Could you check a few things on this model? Use its own coordinates, in mm. A direction names the side the tool comes from. Coordinates: 2 decimals unless noted, no trailing zeros. Order: outer loops, then holes, each group sorted by start corner. A loop starts at its lowest first (then second) coordinate and runs counter-clockwise, first axis right, second up. Notation, with made-up numbers: (32.25, 42) -> (43.25, 42) arc R17 cw to (43.25, 71) -> close; hole circle Ø6 at (74.25, -22.75). An arc over 180 degrees is marked (long way). Use a Markdown table: item, result. Add a question column.
1) If we section it at C-C (x = -32): Write out the boundary of the cut face in (y, z), plus the area to 3 significant figures.
2) Which directions (+Z, -Z, +X, -X, +Y, -Y) give clear straight access to the entire face, cutting with the end or side of a thin tool? Please do faces 5 (the flat face through (15, -15, 60)), 6 (the flat face through (-9, -9, -25)), 7 (the cylindrical face through (18.28, 28.67, -42.26)).
3) Will these pins go through, and if not, where does the flat tip stop? pin 1 Ø4 at (x, z) = (-12, 18) entering from -Y; pin 2 Ø4 at (y, z) = (-28.5, 38) entering from +X; pin 3 Ø5 at (x, z) = (20.5, -10) entering from +Y.
4) If we section it at A-A (y = 0): Write out the boundary of the cut face in (x, z).
5) If I drill on L1, parallel to Y at x = 0, z = 21.5; L2, parallel to Y at x = 0, z = -44.5; L3, parallel to Z at x = -3.5, y = 11.5, over which ranges is the centre line in solid material (lowest first)? Write a range as [from, to].
6) If we section it at D-D (y = 23): Write out the boundary of the cut face in (x, z), plus the area to 3 significant figures.
7) Thinking about a two-plate mould opening in Y: for faces 1 (the cylindrical face through (-4.336, -19.524, 16.905)), 2 (the cylindrical face through (18.28, 28.67, 42.74)), 3 (the flat face through (11, -34, -25)), 4 (the cylindrical face through (2.38, -10.74, -42.74)), which applies, +Y half, -Y half, draft (parallel to the pull), parting line (faces both ways), or undercut?
```python
from build123d import *

# Parameters (mm, degrees)
SKETCH_1_R      = 52
SKETCH_1_R_2    = 34
EXTRUDE_1_DEPTH = 25
SKETCH_1_3_R    = 34
SKETCH_1_3_R_2  = 20
EXTRUDE_2_DEPTH = 60
SKETCH_2_R      = 20
SKETCH_2_R_2    = 11
EXTRUDE_3_DEPTH = 35


with BuildPart() as part:
    # 草图1 → 凸台-拉伸1 (new, symmetric)
    with BuildSketch(Plane.XY):
        Circle(SKETCH_1_R)
        Circle(SKETCH_1_R_2, mode=Mode.SUBTRACT)
    extrude(amount=EXTRUDE_1_DEPTH, both=True)

    # 草图1<3> → 凸台-拉伸2 (add, symmetric)
    with BuildSketch(Plane.XY):
        Circle(SKETCH_1_3_R)
        Circle(SKETCH_1_3_R_2, mode=Mode.SUBTRACT)
    extrude(amount=EXTRUDE_2_DEPTH, both=True)

    # 草图2 → 凸台-拉伸3 (add)
    with BuildSketch(Plane(origin=(0, 0, -60), x_dir=(-1, 0, 0), z_dir=(0, 0, -1))):
        Circle(SKETCH_2_R)
        Circle(SKETCH_2_R_2, mode=Mode.SUBTRACT)
    extrude(amount=-EXTRUDE_3_DEPTH)


solid = part.part
```
Answer sheet:
| question | item | result |
|---|---|---|
| 1 | outline | (-40.99, -25) -> (-11.49, -25) -> (-11.49, -60) -> (11.49, -60) -> (11.49, -25) -> (40.99, -25) -> (40.99, 25) -> (11.49, 25) -> (11.49, 60) -> (-11.49, 60) -> (-11.49, 25) -> (-40.99, 25) -> close |
| 1 | area | 5,710 mm2 |
| 2 | face 5 | +Z, +X, -X, +Y, -Y |
| 2 | face 6 | +Z |
| 2 | face 7 | -Z |
| 3 | pin 1 | y = -51.03 |
| 3 | pin 2 | x = 21.3 |
| 3 | pin 3 | y = 48.79 |
| 4 | outline | (-52, -25) -> (-34, -25) -> (-34, -60) -> (-11, -60) -> (-11, -25) -> (-20, -25) -> (-20, 60) -> (-34, 60) -> (-34, 25) -> (-52, 25) -> close; (11, -60) -> (34, -60) -> (34, -25) -> (52, -25) -> (52, 25) -> (34, 25) -> (34, 60) -> (20, 60) -> (20, -25) -> (11, -25) -> close |
| 5 | L1 | [-52, -20], [20, 52] |
| 5 | L2 | [-34, -11], [11, 34] |
| 5 | L3 | [-60, -25] |
| 6 | outline | (-46.64, -25) -> (-25.04, -25) -> (-25.04, -60) -> (25.04, -60) -> (25.04, -25) -> (46.64, -25) -> (46.64, 25) -> (25.04, 25) -> (25.04, 60) -> (-25.04, 60) -> (-25.04, 25) -> (-46.64, 25) -> close |
| 6 | area | 8,170 mm2 |
| 7 | face 1 | undercut |
| 7 | face 2 | parting line |
| 7 | face 3 | draft |
| 7 | face 4 | undercut |
